```python
from build123d import *

# Parameters (mm, degrees)
SKETCH1_W                      = 40
SKETCH1_H                      = 102
BOSS_EXTRUDE1_DEPTH            = 30
SHELL1_T                       = -2
CUT_EXTRUDE1_REACH             = 95.252
SKETCH2_R                      = 11.43
BOSS_EXTRUDE2_START            = 20
SKETCH3_R                      = 12.7
SKETCH3_R_2                    = 11.43
BOSS_EXTRUDE2_DEPTH            = 20
CUT_EXTRUDE2_REACH             = 95.252
CUT_EXTRUDE2_DIRECTION_2_REACH = 95.252
LPATTERN1_COUNT                = 3
LPATTERN1_PITCH                = 35
SKETCH5_R                      = 16
SKETCH5_R_2                    = 13.7
BOSS_EXTRUDE3_DEPTH            = 2
FILLET1_R                      = 2
CUT_EXTRUDE3_REACH             = 110.185
SKETCH6_R                      = 6.35
BOSS_EXTRUDE4_START            = 5
SKETCH7_R                      = 7.35
SKETCH7_R_2                    = 6.35
BOSS_EXTRUDE4_DEPTH            = 5
FILLET6_R                      = 9


with BuildPart() as part:
    # Sketch1 → Boss-Extrude1 (new body)
    with BuildSketch(Plane(origin=(0, 0, 0), x_dir=(0, 0, -1), z_dir=(1, 0, 0))):
        with Locations((0, 35)):
            Rectangle(SKETCH1_W, SKETCH1_H)
    extrude(amount=BOSS_EXTRUDE1_DEPTH)

    # Shell1
    shell1_openings = [part.faces().sort_by_distance(p)[0] for p in [
        (30, 35, 0),
    ]]
    offset(amount=SHELL1_T, openings=shell1_openings, kind=Kind.INTERSECTION)

    # Sketch2 → Cut-Extrude1 (cut, up to next)
    with BuildSketch(Plane.ZY, mode=Mode.PRIVATE) as cut_extrude1_sk1:
        Circle(SKETCH2_R)
    cut_extrude1_tool1 = extrude(cut_extrude1_sk1.sketch, amount=-CUT_EXTRUDE1_REACH, mode=Mode.PRIVATE) & part.part
    # Sketch2 → Cut-Extrude1 (cut, up to next)
    with BuildSketch(Plane.ZY, mode=Mode.PRIVATE) as cut_extrude1_sk2:
        with Locations((0, 35)):
            Circle(SKETCH2_R)
    cut_extrude1_tool2 = extrude(cut_extrude1_sk2.sketch, amount=-CUT_EXTRUDE1_REACH, mode=Mode.PRIVATE) & part.part
    # Sketch2 → Cut-Extrude1 (cut, up to next)
    with BuildSketch(Plane.ZY, mode=Mode.PRIVATE) as cut_extrude1_sk3:
        with Locations((0, 70)):
            Circle(SKETCH2_R)
    cut_extrude1_tool3 = extrude(cut_extrude1_sk3.sketch, amount=-CUT_EXTRUDE1_REACH, mode=Mode.PRIVATE) & part.part
    add(cut_extrude1_tool1.solids().sort_by_distance((0, 0, 0))[0], mode=Mode.SUBTRACT)
    add(cut_extrude1_tool2.solids().sort_by_distance((0, 35, 0))[0], mode=Mode.SUBTRACT)
    add(cut_extrude1_tool3.solids().sort_by_distance((0, 70, 0))[0], mode=Mode.SUBTRACT)

    # Sketch3 → Boss-Extrude2 (add)
    # profile 1 of 3: a face of its own
    with BuildSketch(Plane.ZY.offset(BOSS_EXTRUDE2_START)):
        Circle(SKETCH3_R)
        Circle(SKETCH3_R_2, mode=Mode.SUBTRACT)
    # profile 2 of 3: a face of its own
    with BuildSketch(Plane.ZY.offset(BOSS_EXTRUDE2_START)):
        with Locations((0, 35)):
            Circle(SKETCH3_R)
        with Locations((0, 35)):
            Circle(SKETCH3_R_2, mode=Mode.SUBTRACT)
    # profile 3 of 3: a face of its own
    with BuildSketch(Plane.ZY.offset(BOSS_EXTRUDE2_START)):
        with Locations((0, 70)):
            Circle(SKETCH3_R)
        with Locations((0, 70)):
            Circle(SKETCH3_R_2, mode=Mode.SUBTRACT)
    extrude(amount=-BOSS_EXTRUDE2_DEPTH)

    # Sketch4 → Cut-Extrude2 (cut, up to next)
    with BuildSketch(Plane.XY, mode=Mode.PRIVATE) as cut_extrude2_sk1:
        with BuildLine():
            ThreePointArc((-20, 82.7), (-18.317957439, 75.380446755), (-13.811148901, 69.372634868))
            Line((-13.811148901, 69.372634868), (0, 57.3))
            Line((0, 57.3), (-20, 57.3))
            Line((-20, 57.3), (-20, 82.7))
        make_face()
    cut_extrude2_tool1 = extrude(cut_extrude2_sk1.sketch, amount=-CUT_EXTRUDE2_REACH, mode=Mode.PRIVATE) & part.part
    cut_extrude2 = cut_extrude2_tool1.solids().sort_by_distance((-13.600187, 63.733143, 0))[0]
    add(cut_extrude2, mode=Mode.SUBTRACT)

    # Sketch4 → Cut-Extrude2 direction 2 (cut, up to next)
    with BuildSketch(Plane.XY, mode=Mode.PRIVATE) as cut_extrude2_direction_2_sk1:
        with BuildLine():
            ThreePointArc((-20, 82.7), (-18.317957439, 75.380446755), (-13.811148901, 69.372634868))
            Line((-13.811148901, 69.372634868), (0, 57.3))
            Line((0, 57.3), (-20, 57.3))
            Line((-20, 57.3), (-20, 82.7))
        make_face()
    cut_extrude2_direction_2_tool1 = extrude(cut_extrude2_direction_2_sk1.sketch, amount=CUT_EXTRUDE2_DIRECTION_2_REACH, mode=Mode.PRIVATE) & part.part
    cut_extrude2_direction_2 = cut_extrude2_direction_2_tool1.solids().sort_by_distance((-13.600187, 63.733143, 0))[0]
    add(cut_extrude2_direction_2, mode=Mode.SUBTRACT)

    # LPattern1: Cut-Extrude2, Cut-Extrude2 direction 2 ×3
    with Locations(*[(0, -i * LPATTERN1_PITCH, 0) for i in range(1, LPATTERN1_COUNT)]):
        add(cut_extrude2, mode=Mode.SUBTRACT)
        add(cut_extrude2_direction_2, mode=Mode.SUBTRACT)

    # Sketch5 → Boss-Extrude3 (add)
    # profile 1 of 3: a face of its own
    with BuildSketch(Plane(origin=(2, 0, 0), x_dir=(0, 0, -1), z_dir=(1, 0, 0))):
        with Locations((0, 70)):
            Circle(SKETCH5_R)
        with Locations((0, 70)):
            Circle(SKETCH5_R_2, mode=Mode.SUBTRACT)
    # profile 2 of 3: a face of its own
    with BuildSketch(Plane(origin=(2, 0, 0), x_dir=(0, 0, -1), z_dir=(1, 0, 0))):
        with Locations(Location((0, 35, 0), (0, 0, 180))):
            Circle(SKETCH5_R)
        with Locations((0, 35)):
            Circle(SKETCH5_R_2, mode=Mode.SUBTRACT)
    # profile 3 of 3: a face of its own
    with BuildSketch(Plane(origin=(2, 0, 0), x_dir=(0, 0, -1), z_dir=(1, 0, 0))):
        Circle(SKETCH5_R)
        Circle(SKETCH5_R_2, mode=Mode.SUBTRACT)
    extrude(amount=BOSS_EXTRUDE3_DEPTH)

    # Fillet1
    fillet1_edges = [part.edges().sort_by_distance(p)[0] for p in [
        (15, 86, 20),
        (15, -16, 20),
        (15, -16, -20),
        (15, 86, -20),
    ]]
    fillet(fillet1_edges, radius=FILLET1_R)

    # Sketch6 → Cut-Extrude3 (cut, up to next)
    with BuildSketch(Plane.XZ.offset(16), mode=Mode.PRIVATE) as cut_extrude3_sk1:
        with Locations(Location((15, 0, 0), (0, 0, 270))):
            Circle(SKETCH6_R)
    cut_extrude3_tool1 = extrude(cut_extrude3_sk1.sketch, amount=-CUT_EXTRUDE3_REACH, mode=Mode.PRIVATE) & part.part
    add(cut_extrude3_tool1.solids().sort_by_distance((15, -16, 0))[0], mode=Mode.SUBTRACT)

    # Sketch7 → Boss-Extrude4 (add)
    with BuildSketch(Plane.XZ.offset(16).offset(BOSS_EXTRUDE4_START)):
        with Locations(Location((15, 0, 0), (0, 0, 90))):
            Circle(SKETCH7_R)
        with Locations(Location((15, 0, 0), (0, 0, 270))):
            Circle(SKETCH7_R_2, mode=Mode.SUBTRACT)
    extrude(amount=-BOSS_EXTRUDE4_DEPTH)

    # Fillet6
    fillet6_edges = [part.edges().sort_by_distance(p)[0] for p in [
        (16, 84, -18),
        (16, 84, 18),
        (16, -14, 18),
        (16, -14, -18),
    ]]
    fillet(fillet6_edges, radius=FILLET6_R)


solid = part.part
```
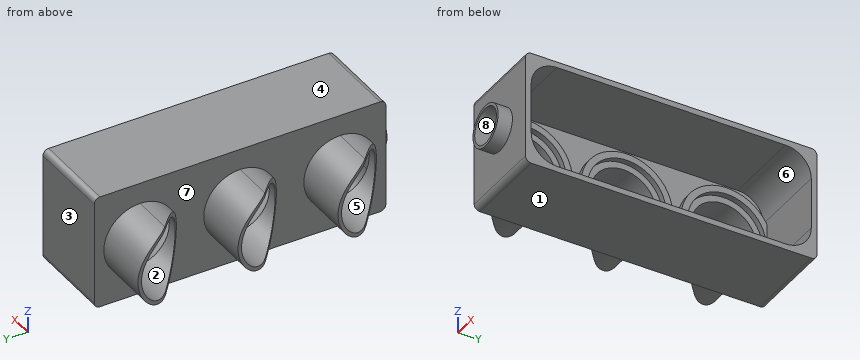
CAD build for the part. Positions are in the model's coordinates, mm. Face numbers are marked on the shaded views. A direction names the side the tool comes from. Round coordinates to 2 decimals unless told otherwise and drop trailing zeros. Write each loop counter-clockwise with the first axis right and the second up, starting at its lowest first coordinate (ties: lowest second). Pieces come first, ordered by that corner, then holes. Notation, with made-up numbers: (8.5, 67.5) -> (15.5, 67.5) arc R10 cw to (15.5, 83.5) -> close; hole circle Ø6 at (-39.5, 82). An arc over 180 degrees is marked (long way). Answer in a Markdown table with one row per item. Add a question column.
Item 1: Mould opens along Z. For the marked faces 1, 2 and 3 say: pulls with the +Z half, pulls with the -Z half, needs draft (parallel to the pull), parting line crosses it, or undercut.
Item 2: Saw through at A-A, the plane x = -7. Write the cut outline in (y, z).
Item 3: Which spindle directions (+Z, -Z, +X, -X, +Y, -Y) get a long thin tool onto all of the face, cutting with end or side? Do the marked faces 4, 5, 6, 7 and 8. Say none if no direction does.
Item 4: Saw through at D-D, the plane y = 32. Write the cut outline in (x, z), then the cut area to 3 significant figures.
Item 5: Drill centre lines: line 1 (Y direction, x = 6, z = 6.5); line 2 (Z direction, x = 28, y = -1.5); line 3 (Z direction, x = -6.75, y = 35). Where is each one in solid material? Low to high. Write a range as from..to.
Item 6: Saw through at B-B, the plane x = 15. Write the cut outline in (y, z), then the cut area to 3 significant figures.
Item 7: Saw through at C-C, the plane y = 3. Write the cut outline in (x, z), then the cut area to 3 significant figures.
Item 8: Drop flat-ended pins along their axis: pin 1 Ø10 at (x, z) = (15, 0) entering from -Y; pin 2 Ø20 at (x, z) = (13.5, 0.5) entering from -Y; pin 3 Ø8 at (y, z) = (73, 13.5) entering from -X; pin 4 Ø11 at (y, z) = (42.5, 4.5) entering from +X. Give the stop position or say it passes through.
Findings below:
| question | item | result |
|---|---|---|
| 1 | face 1 | pulls with the -Z half |
| 1 | face 2 | undercut |
| 1 | face 3 | needs draft |
| 2 | outline | (-6.58, -10.86) arc R12.7 ccw (long way) to (-6.58, 10.86) -> (-6.58, 9.35) arc R11.43 cw (long way) to (-6.58, -9.35) -> close; (28.42, -10.86) arc R12.7 ccw (long way) to (28.42, 10.86) -> (28.42, 9.35) arc R11.43 cw (long way) to (28.42, -9.35) -> close; (63.42, -10.86) arc R12.7 ccw (long way) to (63.42, 10.86) -> (63.42, 9.35) arc R11.43 cw (long way) to (63.42, -9.35) -> close |
| 3 | face 4 | +Z, +X, -X, +Y, -Y |
| 3 | face 5 | +X, -X |
| 3 | face 6 | +X |
| 3 | face 7 | -X |
| 3 | face 8 | -Y |
| 4 | outline | (-11.1, -12.34) -> (0, -12.34) -> (0, -20) -> (30, -20) -> (30, -18) -> (2, -18) -> (2, -15.72) -> (4, -15.72) -> (4, -13.37) -> (2, -13.37) -> (2, -11.03) -> (-11.1, -11.03) -> close; (-11.1, 11.03) -> (2, 11.03) -> (2, 13.37) -> (4, 13.37) -> (4, 15.72) -> (2, 15.72) -> (2, 18) -> (30, 18) -> (30, 20) -> (0, 20) -> (0, 12.34) -> (-11.1, 12.34) -> close |
| 4 | area | 186 mm^2 |
| 5 | line 1 | y = -16..-14, 84..86 |
| 5 | line 2 | z = -20..-18, 18..20 |
| 5 | line 3 | z = -12.7..-11.43, 11.43..12.7 |
| 6 | outline | (-21, -7.35) -> (-16, -7.35) -> (-16, -18) arc R2 ccw to (-14, -20) -> (84, -20) arc R2 ccw to (86, -18) -> (86, 18) arc R2 ccw to (84, 20) -> (-14, 20) arc R2 ccw to (-16, 18) -> (-16, 7.35) -> (-21, 7.35) -> (-21, 6.35) -> (-14, 6.35) -> (-14, 9) arc R9 cw to (-5, 18) -> (75, 18) arc R9 cw to (84, 9) -> (84, -9) arc R9 cw to (75, -18) -> (-5, -18) arc R9 cw to (-14, -9) -> (-14, -6.35) -> (-21, -6.35) -> close |
| 6 | area | 603 mm^2 |
| 7 | outline | (-16.99, -12.34) -> (0, -12.34) -> (0, -20) -> (30, -20) -> (30, -18) -> (2, -18) -> (2, -15.72) -> (4, -15.72) -> (4, -13.37) -> (2, -13.37) -> (2, -11.03) -> (-16.99, -11.03) -> close; (-16.99, 11.03) -> (2, 11.03) -> (2, 13.37) -> (4, 13.37) -> (4, 15.72) -> (2, 15.72) -> (2, 18) -> (30, 18) -> (30, 20) -> (0, 20) -> (0, 12.34) -> (-16.99, 12.34) -> close |
| 7 | area | 202 mm^2 |
| 8 | pin 1 | stops at y = 84 |
| 8 | pin 2 | stops at y = -21 |
| 8 | pin 3 | stops at x = -18.67 |
| 8 | pin 4 | stops at x = 4 |
